Read the model definition and answer for the solid it produces. Units are mm, in the model's axes. A direction names the side the tool comes from. Round coordinates to 2 decimals unless told otherwise and drop trailing zeros. Write each loop counter-clockwise with the first axis right and the second up, starting at its lowest first coordinate (ties: lowest second). Pieces come first, ordered by that corner, then holes. Notation, with made-up numbers: (87, -17) -> (134, -17) arc R24 cw to (134, -3) -> close; hole circle Ø2 at (-19, 79.5). An arc over 180 degrees is marked (long way). Return JSON: item names as keys, results as strings. Group by question number.
(1) Given pin 1 (10 mm diameter, centred on x = -1.5, z = 25.5, fed in from -Y), flat-ended and moving along its own axis, determine where the tip first touches the part or whether it passes through.
(2) A cutting plane is placed at A-A on x = 0. Give the vertices of the cut face in (y, z), then the cut area to 4 significant figures.
(3) Straight lines are drawn through the part: line 1 (Z direction, x = -30, y = 1.45); line 2 (Z direction, x = 0, y = 1.3); line 3 (Z direction, x = -10.5, y = 2.5). For each, find the intervals that lie inside material, in ascending order.
(4) A cutting plane is placed at C-C on x = -30. Give the vertices of the cut face in (y, z), then the cut area to 4 significant figures.
(5) A cutting plane is placed at D-D on y = 0.8. Give the vertices of the cut face in (x, z), then the cut area to 3 significant figures.
(6) For faces 5 (the flat face through (-8.5, 1, 7)), 6 (the flat face through (-15, 3, 29)), determine the directions among +Z, -Z, +X, -X, +Y, -Y from which every point of the face is accessible in a straight line to the end or side of a thin tool.
(7) The mould has two halves that part along Z. Classify faces 1 (the cylindrical face through (5.35, 1.52, 62.64)), 2 (the cylindrical face through (-0.867, 1.479, -3.905)), 3 (the flat face through (-15, 1, 0.25)), 4 (the cylindrical face through (-35.39, 1.52, -6.1)): released by +Z, released by -Z, zero draft, split by the parting line, or undercut.
(8) A cutting plane is placed at B-B on z = 57.5. Give the vertices of the cut face in (x, y).
```python
from build123d import *

# Parameters (mm, degrees)
F0_W     = 42.5
F0_H     = 70.5
F0_R     = 2.5
F0_W_2   = 13
F0_H_2   = 13
F0_R_2   = 4
F1_DEPTH = 3
F2_R     = 3


with BuildPart() as f1:
    # F0 (on Front) → F1 (new body)
    with BuildSketch(Plane.XZ):
        with Locations((-15, 28.25)):
            Rectangle(F0_W, F0_H)
        with Locations((-30, 19.5)):
            Circle(F0_R, mode=Mode.SUBTRACT)
        with Locations((-15, 6.75)):
            Rectangle(F0_W_2, F0_H_2, mode=Mode.SUBTRACT)
        Circle(F0_R_2, mode=Mode.SUBTRACT)
        with Locations((0, 19.5)):
            Circle(F0_R, mode=Mode.SUBTRACT)
        with Locations((-30, 57.5)):
            Circle(F0_R, mode=Mode.SUBTRACT)
        with Locations((0, 57.5)):
            Circle(F0_R, mode=Mode.SUBTRACT)
    extrude(amount=-F1_DEPTH)

    # F2
    f2_edges = [f1.edges().sort_by_distance(p)[0] for p in [
        (-36.25, 1.5, 63.5),
        (6.25, 1.5, 63.5),
        (6.25, 1.5, -7),
        (-36.25, 1.5, -7),
    ]]
    fillet(f2_edges, radius=F2_R)


solid = f1.part
```
Checks:
{
 "1": {"pin 1": "stops at y = 0"},
 "2": {"outline": "(0, -7) -> (3, -7) -> (3, -4) -> (0, -4) -> close; (0, 4) -> (3, 4) -> (3, 17) -> (0, 17) -> close; (0, 22) -> (3, 22) -> (3, 55) -> (0, 55) -> close; (0, 60) -> (3, 60) -> (3, 63.5) -> (0, 63.5) -> close", "area": "157.5 mm^2"},
 "3": {"line 1": "z = -7 to 17, 22 to 55, 60 to 63.5", "line 2": "z = -7 to -4, 4 to 17, 22 to 55, 60 to 63.5", "line 3": "z = -7 to 0.25, 13.25 to 63.5"},
 "4": {"outline": "(0, -7) -> (3, -7) -> (3, 17) -> (0, 17) -> close; (0, 22) -> (3, 22) -> (3, 55) -> (0, 55) -> close; (0, 60) -> (3, 60) -> (3, 63.5) -> (0, 63.5) -> close", "area": "181.5 mm^2"},
 "5": {"outline": "(-36.25, -4) arc R3 ccw to (-33.25, -7) -> (3.25, -7) arc R3 ccw to (6.25, -4) -> (6.25, 60.5) arc R3 ccw to (3.25, 63.5) -> (-33.25, 63.5) arc R3 ccw to (-36.25, 60.5) -> close; hole circle Ø5 at (-30, 19.5); hole circle Ø5 at (-30, 57.5); hole (-21.5, 0.25) -> (-8.5, 0.25) -> (-8.5, 13.25) -> (-21.5, 13.25) -> close; hole circle Ø8 at (0, 0); hole circle Ø5 at (0, 19.5); hole circle Ø5 at (0, 57.5)", "area": "2,690 mm^2"},
 "6": {"face 5": "+Y, -Y", "face 6": "+Z, -Z, +X, -X, +Y"},
 "7": {"face 1": "released by +Z", "face 2": "undercut", "face 3": "undercut", "face 4": "released by -Z"},
 "8": {"outline": "(-36.25, 0) -> (-32.5, 0) -> (-32.5, 3) -> (-36.25, 3) -> close; (-27.5, 0) -> (-2.5, 0) -> (-2.5, 3) -> (-27.5, 3) -> close; (2.5, 0) -> (6.25, 0) -> (6.25, 3) -> (2.5, 3) -> close"}
}
